For this review, use the dimensioned drawing (mm, ordinates from the lowest corner) and the shaded views. A direction names the side the tool comes from. Round coordinates to 2 decimals unless told otherwise and drop trailing zeros. Loops run counter-clockwise (first coordinate to the right, second up) from the corner with the lowest first, then second, coordinate; pieces in that order, holes last. Notation, with made-up numbers: (42.25, 73) - (71.25, 73) arc R23 ccw to (71.25, 85) - close; hole circle Ø6 at (37.25, 27). An arc over 180 degrees is marked (long way). Use one line per item in the form item = value. Start each with the question number.
(1) We need section C-C, the plane x = 71.5. Write out the cut boundary in (y, z), then the cut area to 3 significant figures.
(2) The part is to be moulded in two halves that separate along X. For the marked faces 1, 2, 3 and 4, say which applies: released by +X, released by -X, zero draft, split by the parting line, or undercut.
(3) We need section D-D, the plane y = 31. Write out the cut boundary in (x, z).
(4) Wall thickness on probe 1 along Y at (x, z) = (4, 5.25); probe 2 along Y at (x, z) = (40.5, 5.5); probe 3 along Y at (x, z) = (10.5, 7): over which ranges is each line inside the solid? List them lowest first. Write a range as [from, to].
(5) We need section B-B, the plane z = 13.5. Write out the cut boundary in (x, y).
(6) We need section A-A, the plane y = 46.5. Write out the cut boundary in (x, z).
(7) Machinability: for the marked faces 5, 6 and 7, which of the approach directions +Z, -Z, +X, -X, +Y, -Y give a long, thin tool a straight path to every point of the face, cutting with its end or side? Answer none if there is none.
(8) For pin 1 (10 mm diameter, centred on x = 31.5, z = 18.5, fed in from +Y); pin 2 (3.5 mm diameter, centred on y = 20, z = 10, fed in from +X); pin 3 (12 mm diameter, centred on x = 17.5, z = 7, fed in from -Y), all flat-tipped, find the tip position at first contact; note any pin that passes through.
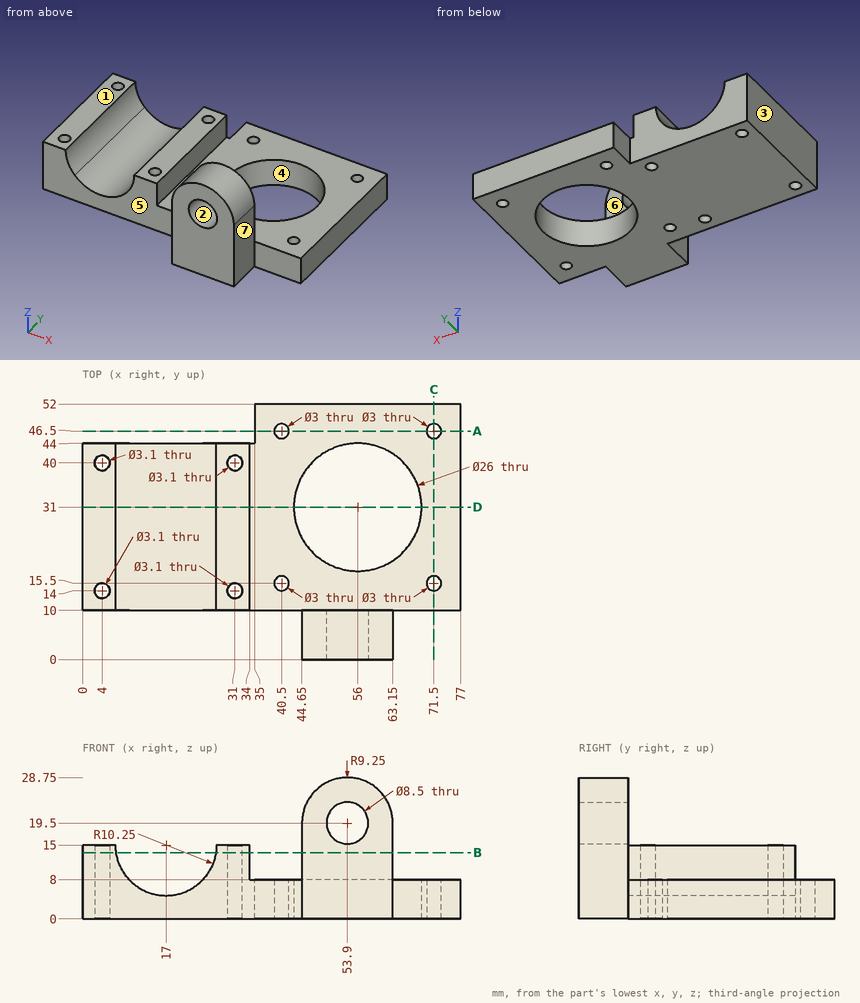
Data:
q1.outline = (10, 0) - (14, 0) - (14, 8) - (10, 8) - close; (17, 0) - (45, 0) - (45, 8) - (17, 8) - close; (48, 0) - (52, 0) - (52, 8) - (48, 8) - close
q1.area = 288 mm^2
q2.face_1 = zero draft
q2.face_2 = undercut
q2.face_3 = released by -X
q2.face_4 = undercut
q3.outline = (0, 0) - (43, 0) - (43, 8) - (34, 8) - (34, 15) - (27.25, 15) arc R10.25 cw to (6.75, 15) - (0, 15) - close; (69, 0) - (77, 0) - (77, 8) - (69, 8) - close
q4.probe_1 = [10, 12.45], [15.55, 38.45], [41.55, 44]
q4.probe_2 = [10, 14], [17, 45], [48, 52]
q4.probe_3 = [10, 44]
q5.outline = (0, 10) - (6.86, 10) - (6.86, 44) - (0, 44) - close; (27.14, 10) - (34, 10) - (34, 44) - (27.14, 44) - close; (44.65, 0) - (63.15, 0) - (63.15, 10) - (44.65, 10) - close; hole circle Ø3.1 at (4, 14); hole circle Ø3.1 at (4, 40); hole circle Ø3.1 at (31, 14); hole circle Ø3.1 at (31, 40)
q6.outline = (35, 0) - (39, 0) - (39, 8) - (35, 8) - close; (42, 0) - (70, 0) - (70, 8) - (42, 8) - close; (73, 0) - (77, 0) - (77, 8) - (73, 8) - close
q7.face_5 = +Z, -Z, -X, -Y
q7.face_6 = +Z, +X, +Y
q7.face_7 = +Z, -Z, +X, -Y
q8.pin_1 = 44
q8.pin_2 = 34
q8.pin_3 = 10
